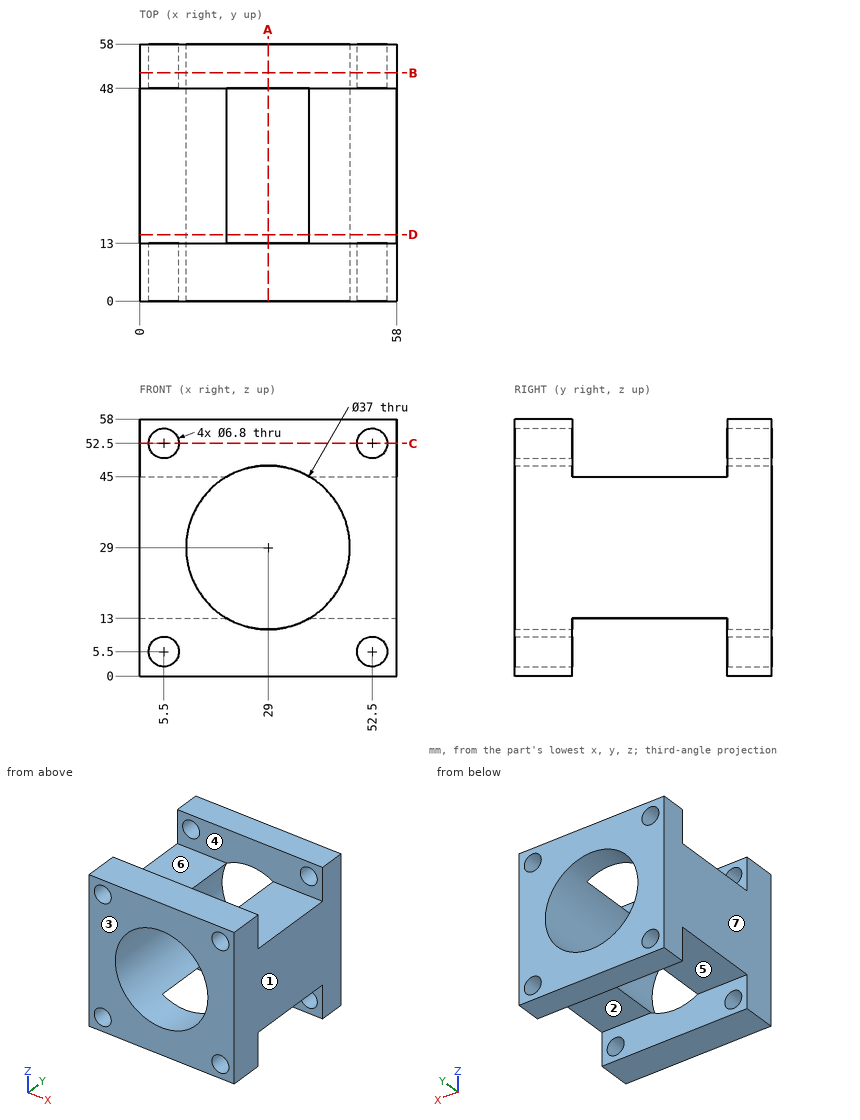
Verification items for this drawing (mm, ordinates from the low corner). A direction names the side the tool comes from. Give positions to 0.01 mm unless a question says otherwise; leave off trailing zeros. Order: outer loops, then holes, each group sorted by start corner. A loop starts at its lowest first (then second) coordinate and runs counter-clockwise, first axis right, second up. Notation, with made-up numbers: M 87,50.25 L 141,50.25 A13 cw 141,59.25 Z; hole C 3,87 d11. An arc over 180 degrees is marked long. Use a Markdown table: item, result.
Item 1: Material ranges on line 1 along Z through (x, y) = (52.5, 4); line 2 along Z through (x, y) = (51, 50); line 3 along Y through (x, z) = (37, 9), recorded low to high.
Answers follow:
| item | result |
|---|---|
| line 1 | z = 0 to 2.1, 8.9 to 49.1, 55.9 to 58 |
| line 2 | z = 0 to 2.45, 8.55 to 49.45, 55.55 to 58 |
| line 3 | y = 0 to 13, 48 to 58 |
Item 2: Section check D-D (y = 15). Record the cut outline in (x, z), and give its area (3 significant figures).
Answers follow:
| item | result |
|---|---|
| outline | M 0,13 L 19.71,13 A18.5 cw 19.71,45 L 0,45 Z; M 38.29,13 L 58,13 L 58,45 L 38.29,45 A18.5 cw Z |
| area | 844 mm2 |
Item 3: Section check A-A (x = 29). Record the cut outline in (y, z).
Answers follow:
| item | result |
|---|---|
| outline | M 0,0 L 13,0 L 13,10.5 L 0,10.5 Z; M 0,47.5 L 13,47.5 L 13,58 L 0,58 Z; M 48,0 L 58,0 L 58,10.5 L 48,10.5 Z; M 48,47.5 L 58,47.5 L 58,58 L 48,58 Z |
Item 4: Section check C-C (z = 52.5). Record the cut outline in (x, y), and give its area (3 significant figures).
Answers follow:
| item | result |
|---|---|
| outline | M 0,0 L 2.1,0 L 2.1,13 L 0,13 Z; M 0,48 L 2.1,48 L 2.1,58 L 0,58 Z; M 8.9,0 L 49.1,0 L 49.1,13 L 8.9,13 Z; M 8.9,48 L 49.1,48 L 49.1,58 L 8.9,58 Z; M 55.9,0 L 58,0 L 58,13 L 55.9,13 Z; M 55.9,48 L 58,48 L 58,58 L 55.9,58 Z |
| area | 1,020 mm2 |
Item 5: Draft check along Y on the marked faces 1, 2, 3 and 4. Enter one of: +Y half, -Y half, draft (parallel to the pull), parting line (faces both ways), or undercut.
Answers follow:
| item | result |
|---|---|
| face 1 | draft |
| face 2 | undercut |
| face 3 | -Y half |
| face 4 | undercut |
Item 6: Tool access check on the marked faces 5, 6 and 7. Record the directions out of +Z, -Z, +X, -X, +Y, -Y that give a thin tool (end or side, any length) a straight path to the whole face; none if there is none.
Answers follow:
| item | result |
|---|---|
| face 5 | -Z, +X, -X |
| face 6 | +Z, +X, -X |
| face 7 | +Z, -Z, -X, +Y, -Y |
Item 7: Depth check by flat-ended pin: P1, Ø6.5, axis at x = 33, z = 52.5, coming from the -Y side; P2, Ø2, axis at x = 42, y = 20.5, coming from the +Z side; P3, Ø6, axis at x = 46, y = 31, coming from the -Z side. Enter the tip coordinate at first touch or a pass-through.
Answers follow:
| item | result |
|---|---|
| P1 | stops at y = 0 |
| P2 | stops at z = 45 |
| P3 | stops at z = 13 |
Item 8: Section check B-B (y = 51.5). Record the cut outline in (x, z), and give its area (3 significant figures).
Answers follow:
| item | result |
|---|---|
| outline | M 0,0 L 58,0 L 58,58 L 0,58 Z; hole C 5.5,5.5 d6.8; hole C 5.5,52.5 d6.8; hole C 29,29 d37; hole C 52.5,5.5 d6.8; hole C 52.5,52.5 d6.8 |
| area | 2,140 mm2 |
